Read the model definition and answer for the solid it produces. Units are mm, in the model's axes. A direction names the side the tool comes from. Coordinates: 2 decimals unless noted, no trailing zeros. Loops run counter-clockwise (first coordinate to the right, second up) from the corner with the lowest first, then second, coordinate; pieces in that order, holes last.
from build123d import *

# Parameters (mm, degrees)
SKETCH001_W  = 29.6
SKETCH001_H  = 21.7
PAD001_DEPTH = 15
SKETCH003_R  = 13.9
PAD002_DEPTH = 7.9
SKETCH004_R  = 1.5
POCKET_DEPTH = 15.001


with BuildPart() as part:
    # Sketch001 → Pad001 (new body, symmetric)
    with BuildSketch(Plane.XY):
        with Locations((0, -10.85)):
            Rectangle(SKETCH001_W, SKETCH001_H)
    extrude(amount=PAD001_DEPTH, both=True)

    # Sketch003 → Pad002 (join)
    with BuildSketch(Plane.XZ):
        Circle(SKETCH003_R)
    extrude(amount=-PAD002_DEPTH)

    # Sketch004 → Pocket (cut, through all)
    with BuildSketch(Plane.XY):
        with Locations((-10, -5.1)):
            Circle(SKETCH004_R)
        with Locations((10, -5.1)):
            Circle(SKETCH004_R)
    extrude(amount=-POCKET_DEPTH, mode=Mode.SUBTRACT)


solid = part.part
Q1. Straight lines are drawn through the part: probe 1 along Y at (x, z) = (10, -5); probe 2 along X at (y, z) = (4.75, -11); probe 3 along Y at (x, z) = (8.75, -7.25). For each, find the intervals that lie inside material, in ascending order.
Findings below:
probe 1: y = -21.7 to -6.6, -3.6 to 7.9
probe 2: x = -8.5 to 8.5
probe 3: y = -21.7 to -5.93, -4.27 to 7.9
Q2. A cutting plane is placed at B-B (x = 0). Give the vertices of the cut face in (y, z), then the cut area to 3 significant figures.
Findings below:
outline: (-21.7, -15) - (0, -15) - (0, -13.9) - (7.9, -13.9) - (7.9, 13.9) - (0, 13.9) - (0, 15) - (-21.7, 15) - close
area: 871 mm2
Q3. Which of the six approach directions +Z, -Z, +X, -X, +Y, -Y give full straight-line access (tool end or side, diameter ignored) to faces 1 (the face through (-11, 0, 9)), 2 (the face through (-10, -5, 0)), 3 (the face through (-14.8, -11, 0))?
Findings below:
face 1: +Y
face 2: -Z
face 3: +Z, -Z, -X, +Y, -Y
Q4. Determine the mould class of faces 4 (the face through (8.5, -5.03, -7.4)), 5 (the face through (0, -21.7, 0)), 6 (the face through (14.8, -11, 0)) for opening direction Y: +Y half, -Y half, draft (parallel to the pull), parting line (faces both ways), or undercut.
Findings below:
face 4: undercut
face 5: -Y half
face 6: draft
Q5. A cutting plane is placed at A-A (y = -5.1). Give the vertices of the cut face in (x, z), then the cut area to 3 significant figures.
Findings below:
outline: (-14.8, -15) - (-11.5, -15) - (-11.5, 0) - (-8.5, 0) - (-8.5, -15) - (8.5, -15) - (8.5, 0) - (11.5, 0) - (11.5, -15) - (14.8, -15) - (14.8, 15) - (-14.8, 15) - close
area: 798 mm2
Q6. A cutting plane is placed at C-C (z = 4.75). Give the vertices of the cut face in (x, y), then the cut area to 3 significant figures.
Findings below:
outline: (-14.8, -21.7) - (14.8, -21.7) - (14.8, 0) - (13.06, 0) - (13.06, 7.9) - (-13.06, 7.9) - (-13.06, 0) - (-14.8, 0) - close
area: 849 mm2
Q7. A cutting plane is placed at D-D (x = 10). Give the vertices of the cut face in (y, z).
Findings below:
outline: (-21.7, -15) - (-6.6, -15) - (-6.6, 0) - (-3.6, 0) - (-3.6, -15) - (0, -15) - (0, -9.65) - (7.9, -9.65) - (7.9, 9.65) - (0, 9.65) - (0, 15) - (-21.7, 15) - close
Q8. Flat-ended cylindrical pins translate along their axes: pin 1 Ø0.9 at (x, y) = (10.5, -5.5) entering from -Z; pin 2 Ø3 at (y, z) = (3.5, -6.5) entering from +X. Find the tip coordinate at first contact, or state that the pin passes through.
Findings below:
pin 1: stops at z = 0
pin 2: stops at x = 12.97
